from build123d import *

# Parameters (mm, degrees)
SKETCH1_W           = 95
SKETCH1_H           = 8
SKETCH1_R           = 2.58
SKETCH1_R_2         = 2.59
BOSS_EXTRUDE1_DEPTH = 3
REDONDEO2_R         = 4


with BuildPart() as part:
    # Sketch1 → Boss-Extrude1 (new body)
    with BuildSketch(Plane(origin=(0, 0, 0), x_dir=(1, 0, 0), z_dir=(0, 1, 0))):
        with Locations((-0.1, 1.5)):
            Rectangle(SKETCH1_W, SKETCH1_H)
        with Locations(Location((-42.1, 1.5, 0), (0, 0, 270))):
            Circle(SKETCH1_R, mode=Mode.SUBTRACT)
        with Locations(Location((41.9, 1.5, 0), (0, 0, 270))):
            Circle(SKETCH1_R_2, mode=Mode.SUBTRACT)
    extrude(amount=BOSS_EXTRUDE1_DEPTH)

    # Redondeo2
    redondeo2_edges = [part.edges().sort_by_distance(p)[0] for p in [
        (47.4, 1.5, -5.5),
        (47.4, 1.5, 2.5),
        (-47.6, 1.5, -5.5),
        (-47.6, 1.5, 2.5),
    ]]
    fillet(redondeo2_edges, radius=REDONDEO2_R - 0.0001)  # a hair under: the kernel refuses the full size


solid = part.part
The listing builds one solid part. Answer for the finished solid, in the listing's coordinates (mm). Give positions to 0.01 mm unless a question says otherwise; leave off trailing zeros. Write each loop counter-clockwise with the first axis right and the second up, starting at its lowest first coordinate (ties: lowest second). Pieces come first, ordered by that corner, then holes. Notation, with made-up numbers: (38, 37) -> (72, 37) arc R23 cw to (72, 62) -> close; hole circle Ø4 at (-15.75, 33). An arc over 180 degrees is marked (long way). Use a Markdown table: item, result.
(1) Find the intervals of material crossed by probe 1 along X at (y, z) = (2.6, -1.5); probe 2 along X at (y, z) = (2.7, -2); probe 3 along Z at (x, y) = (40, 0.4), in increasing order. Write a range as from..to.
Return value:
| item | result |
|---|---|
| probe 1 | -47.6..-44.68, -39.52..39.31, 44.49..47.4 |
| probe 2 | -47.57..-44.63, -39.57..39.36, 44.44..47.37 |
| probe 3 | -5.5..-3.26, 0.26..2.5 |
(2) Determine the mould class of faces 1 (the cylindrical face through (-39.542, 1.479, -1.836)), 2 (the cylindrical face through (-46.459, 1.521, 1.297)), 3 (the cylindrical face through (46.197, 1.521, -4.359)) for opening direction Z: released by +Z, released by -Z, zero draft, split by the parting line, or undercut.
Return value:
| item | result |
|---|---|
| face 1 | undercut |
| face 2 | released by +Z |
| face 3 | released by -Z |
(3) Section C-C, the plane x = 41.9 is taken. Determine the outline of the cut face in (y, z), then the cut area to 3 significant figures.
Return value:
| item | result |
|---|---|
| outline | (0, -5.5) -> (3, -5.5) -> (3, -4.09) -> (0, -4.09) -> close; (0, 1.09) -> (3, 1.09) -> (3, 2.5) -> (0, 2.5) -> close |
| area | 8.46 mm2 |
(4) Section B-B, the plane y = 2.25 is taken. Give the number of separate pieces and of enclosed holes in the cut face, then the cut area to 3 significant figures.
Return value:
| item | result |
|---|---|
| separate pieces | 1 |
| enclosed holes | 2 |
| area | 704 mm2 |
(5) Section A-A, the plane x = -42.1 is taken. Determine the outline of the cut face in (y, z).
Return value:
| item | result |
|---|---|
| outline | (0, -5.5) -> (3, -5.5) -> (3, -4.08) -> (0, -4.08) -> close; (0, 1.08) -> (3, 1.08) -> (3, 2.5) -> (0, 2.5) -> close |
(6) A flat-ended cylindrical pin translates along its axis: P1, Ø3, axis at x = 41.9, z = -1.5, coming from the -Y side. Find the tip coordinate at first contact, or state that the pin passes through.
Return value:
| item | result |
|---|---|
| P1 | through |
